Autodesk Fusion 360 part; units mm, degrees
sketch "Sketch1" plane through (0, 0, 0) normal (0, 0, 1) x (1, 0, 0)
  line L0 (0, 0) -> (80, 0)
  line L1 (80, 0) -> (80, 100)
  line L2 (80, 100) -> (0, 100)
  line L3 (0, 100) -> (0, 0)
  line L4 (40, 100) -> (40, 130)
  line L5 (40, 130) -> (50, 120)
  line L6 (50, 120) -> (55, 125)
  line L7 (55, 125) -> (65, 115)
  line L8 (65, 115) -> (80, 100)
  line L9 (40, 130) -> (30, 120)
  line L10 (30, 120) -> (25, 125)
  line L11 (25, 125) -> (0, 100)
extrude "Extrude1" add sketch "Sketch1" along normal blind 6
extrude "Extrude2" cut 1 faces at (26.6667, 66.6667, 6) along direction (0, 0, -1) blind 4.4
sketch "Sketch2" plane through (0, 0, 1.6) normal (0, 0, 1) x (-1, 0, 0)
  line L0 (-40, -130) -> (-30, -120)
  line L1 (-30, -120) -> (-25, -125)
  line L2 (-25, -125) -> (0, -100)
  line L3 (0, -100) -> (0, 0)
  line L4 (0, 0) -> (-80, 0)
  line L5 (-80, 0) -> (-80, -100)
  line L6 (-80, -100) -> (-55, -125)
  line L7 (-55, -125) -> (-50, -120)
  line L8 (-50, -120) -> (-40, -130)
  line L9 (-80, -100) -> (0, 0) construction
  line L10 (0, -100) -> (-80, 0) construction
  line L11 (-70, -75) -> (-10, -75) construction
  line L12 (-10, -75) -> (-10, -25) construction
  line L13 (-10, -25) -> (-70, -25) construction
  line L14 (-70, -25) -> (-70, -75) construction
  line L15 (-70, -75) -> (-10, -25) construction
  line L16 (-10, -75) -> (-70, -25) construction
  circle A0 centre (-10, -75) radius 1.65
  circle A1 centre (-70, -75) radius 1.65
  circle A2 centre (-10, -25) radius 1.65
  circle A3 centre (-70, -25) radius 1.65
  point P0 (-40, -50)
  dimension "d5" = 60
  dimension "d6" = 50
  dimension "d7" = 3.3
  dimension "d8" = 3.3
  dimension "d9" = 3.3
  dimension "d10" = 3.3
extrude "Extrude3" cut sketch "Sketch2" against normal blind 55 contours A0 | A1 | A2 | A3
sketch "Sketch3" plane through (0, 0, 1.6) normal (0, 0, 1) x (-1, 0, 0)
  circle A0 centre (-10, -25) radius 1.65
  circle A1 centre (-10, -75) radius 1.65
  circle A2 centre (-70, -25) radius 1.65
  circle A3 centre (-70, -75) radius 1.65
  line L0 (-40, -130) -> (-30, -120)
  line L1 (-30, -120) -> (-25, -125)
  line L2 (-25, -125) -> (0, -100)
  line L3 (0, -100) -> (0, 0)
  line L4 (0, 0) -> (-80, 0)
  line L5 (-80, 0) -> (-80, -100)
  line L6 (-80, -100) -> (-55, -125)
  line L7 (-55, -125) -> (-50, -120)
  line L8 (-50, -120) -> (-40, -130)
sketch "Sketch4" plane through (0, 0, 1.6) normal (0, 0, 1) x (1, 0, 0)
Geometry check sheet. Reference: the model listing, model coordinates, mm. A direction names the side the tool comes from. Coordinates: 2 decimals unless noted, no trailing zeros. Loops run counter-clockwise (first coordinate to the right, second up) from the corner with the lowest first, then second, coordinate; pieces in that order, holes last.
Item 1: Sectioned sample at C-C, the plane x = 10. Record the boundary of the cut face in (y, z).
Item 2: Sectioned sample at B-B, the plane y = 25. Record the boundary of the cut face in (x, z).
Item 3: Access from +Z, -Z, +X, -X, +Y, -Y to the whole of each face (thin tool, end or side, straight path). Record for faces 1 (the face through (52, 122, 1)), 2 (the face through (71.65, 74.93, 0.81)).
Item 4: Release check for a two-part mould opening along Y. For faces 3 (the face through (71.216, 23.885, 0.811)), 4 (the face through (35, 125, 1)), 5 (the face through (39, 51, 0)) record: released by +Y, released by -Y, zero draft, split by the parting line, or undercut.
Item 5: Sectioned sample at A-A, the plane z = 0.8. Record the boundary of the cut face in (x, y), then the cut area to 3 significant figures.
Item 6: Sectioned sample at D-D, the plane y = 112. Record the boundary of the cut face in (x, z).
Item 7: Thickness scan on line 1 (X direction, y = 75, z = 0.7); line 2 (Y direction, x = 70, z = 1.15); line 3 (Y direction, x = 71, z = 0.6). Record the ranges inside material, lowest first.
Check result:
1. outline: (0, 0) - (23.35, 0) - (23.35, 1.6) - (0, 1.6) - close; (26.65, 0) - (73.35, 0) - (73.35, 1.6) - (26.65, 1.6) - close; (76.65, 0) - (110, 0) - (110, 1.6) - (76.65, 1.6) - close
2. outline: (0, 0) - (8.35, 0) - (8.35, 1.6) - (0, 1.6) - close; (11.65, 0) - (68.35, 0) - (68.35, 1.6) - (11.65, 1.6) - close; (71.65, 0) - (80, 0) - (80, 1.6) - (71.65, 1.6) - close
3. face 1: +Z, -Z, +Y
3. face 2: +Z, -Z
4. face 3: undercut
4. face 4: released by +Y
4. face 5: zero draft
5. outline: (0, 0) - (80, 0) - (80, 100) - (55, 125) - (50, 120) - (40, 130) - (30, 120) - (25, 125) - (0, 100) - close; hole circle Ø3.3 at (10, 25); hole circle Ø3.3 at (10, 75); hole circle Ø3.3 at (70, 25); hole circle Ø3.3 at (70, 75)
5. area: 9,320 mm2
6. outline: (12, 0) - (68, 0) - (68, 1.6) - (12, 1.6) - close
7. line 1: x = 0 to 8.35, 11.65 to 68.35, 71.65 to 80
7. line 2: y = 0 to 23.35, 26.65 to 73.35, 76.65 to 110
7. line 3: y = 0 to 23.69, 26.31 to 73.69, 76.31 to 109
